Can you work these out from the model? Positions are in its coordinate system, mm. Face numbers are marked on the shaded views. A direction names the side the tool comes from. Coordinates: 2 decimals unless noted, no trailing zeros. Order: outer loops, then holes, each group sorted by start corner. A loop starts at its lowest first (then second) coordinate and runs counter-clockwise, first axis right, second up. Notation, with made-up numbers: (53.5, 14) -> (87.5, 14) arc R11 cw to (87.5, 21) -> close; hole circle Ø5 at (38, -25.75). An arc over 180 degrees is marked (long way). Answer in a Markdown table with one row per item.
```python
from build123d import *

# Parameters (mm, degrees)
S01_80_MM_TYRE_AND_TWO_INWARD_BEAD_LIP_R       = 40
F_01_80_MM_TYRE_AND_TWO_INWARD_BEAD_LIPS_DEPTH = 19.8
F_02_START                                     = 2.1
F_02_CENTRAL_KEYED_DRIVE_RECESS_BETWEEN_DEPTH  = 15.6


with BuildPart() as part:
    # S01 - 80 mm tyre and two inward bead lips → 01 - 80 mm tyre and two inward bead lips (new body)
    with BuildSketch(Plane.XY):
        with Locations(Location((0, 0, 0), (0, 0, 180))):
            Circle(S01_80_MM_TYRE_AND_TWO_INWARD_BEAD_LIP_R)
        Polygon((32.744885511, 8.773965629), (23.970919882, 23.970919882), (8.773965629, 32.744885511), (-8.773965629, 32.744885511), (-23.970919882, 23.970919882), (-32.744885511, 8.773965629), (-32.744885511, -8.773965629), (-23.970919882, -23.970919882), (-8.773965629, -32.744885511), (8.773965629, -32.744885511), (23.970919882, -23.970919882), (32.744885511, -8.773965629), align=None, mode=Mode.SUBTRACT)
    extrude(amount=F_01_80_MM_TYRE_AND_TWO_INWARD_BEAD_LIPS_DEPTH)

    # S02 - Central keyed drive recess between end beads → 02 - Central keyed drive recess between end beads (cut)
    with BuildSketch(Plane.XY.offset(F_02_START)):
        Polygon((33.710811337, 9.032784674), (24.678026663, 24.678026663), (9.032784674, 33.710811337), (-9.032784674, 33.710811337), (-24.678026663, 24.678026663), (-33.710811337, 9.032784674), (-33.710811337, -9.032784674), (-24.678026663, -24.678026663), (-9.032784674, -33.710811337), (9.032784674, -33.710811337), (24.678026663, -24.678026663), (33.710811337, -9.032784674), align=None)
    extrude(amount=F_02_CENTRAL_KEYED_DRIVE_RECESS_BETWEEN_DEPTH, mode=Mode.SUBTRACT)


solid = part.part
```
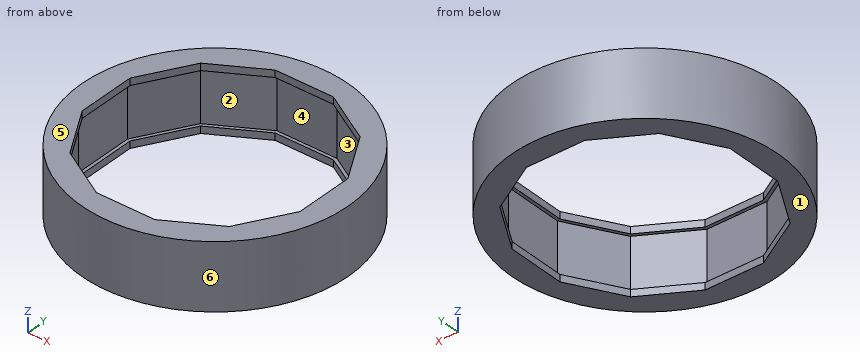
(1) We'd pull the mould along X, two halves only. Please class the marked faces 3, 4, 5 and 6: +X half, -X half, draft (parallel to the pull), parting line (faces both ways), or undercut.
Response values:
| item | result |
|---|---|
| face 3 | undercut |
| face 4 | undercut |
| face 5 | draft |
| face 6 | parting line |
(2) I need wall thicknesses on line 1 (Z direction, x = -33.5, y = -3.5); line 2 (X direction, y = -33, z = 14.5); line 3 (Y direction, x = 31, z = 1). Which ranges of each line are inside material? Lowest first, please. Write a range as [from, to].
Response values:
| item | result |
|---|---|
| line 1 | [0, 2.1], [17.7, 19.8] |
| line 2 | [-22.61, -10.26], [10.26, 22.61] |
| line 3 | [-25.28, -11.8], [11.8, 25.28] |
(3) Will these pins go through, and if not, where does the flat tip stop? pin 1 Ø1.1 at (x, z) = (2, 18.5) entering from -Y; pin 2 Ø20 at (x, y) = (2, -14.5) entering from +Z; pin 3 Ø3 at (x, z) = (25.5, 7) entering from +Y; pin 4 Ø1 at (y, z) = (4.5, 0.5) entering from +X.
Response values:
| item | result |
|---|---|
| pin 1 | y = -39.97 |
| pin 2 | through |
| pin 3 | y = 32 |
| pin 4 | x = 39.8 |
(4) On a 3-axis mill with a long thin cutter (end or side, diameter ignored), from which of +Z, -Z, +X, -X, +Y, -Y can I reach the whole of each face in a straight line? I mean the marked faces 1 and 2. Say none if no direction works.
Response values:
| item | result |
|---|---|
| face 1 | -Z, +X, -X, +Y, -Y |
| face 2 | none |
(5) Suppose I cut it at A-A (x = 0). Please give me the cut outline in (y, z), and give its area (3 significant figures).
Response values:
| item | result |
|---|---|
| outline | (-40, 0) -> (-32.74, 0) -> (-32.74, 2.1) -> (-33.71, 2.1) -> (-33.71, 17.7) -> (-32.74, 17.7) -> (-32.74, 19.8) -> (-40, 19.8) -> close; (32.74, 0) -> (40, 0) -> (40, 19.8) -> (32.74, 19.8) -> (32.74, 17.7) -> (33.71, 17.7) -> (33.71, 2.1) -> (32.74, 2.1) -> close |
| area | 257 mm2 |
(6) Suppose I cut it at C-C (z = 10). Please give me the cut outline in (x, y).
Response values:
| item | result |
|---|---|
| outline | circle Ø80 at (0, 0); hole (-33.71, -9.03) -> (-24.68, -24.68) -> (-9.03, -33.71) -> (9.03, -33.71) -> (24.68, -24.68) -> (33.71, -9.03) -> (33.71, 9.03) -> (24.68, 24.68) -> (9.03, 33.71) -> (-9.03, 33.71) -> (-24.68, 24.68) -> (-33.71, 9.03) -> close |
